from build123d import *

# Parameters (mm, degrees)
SZKIC1_W                    = 58
SZKIC1_H                    = 11
SZKIC1_R                    = 1.55
DODANIE_WYCI_GNI_CIE1_DEPTH = 6


with BuildPart() as part:
    # Szkic1 → Dodanie-wyciągnięcie1 (new body)
    with BuildSketch(Plane.ZY):
        with Locations((-846, 35.19227062)):
            Rectangle(SZKIC1_W, SZKIC1_H)
        with Locations((-869, 36.69227062)):
            Circle(SZKIC1_R, mode=Mode.SUBTRACT)
        with Locations((-821, 36.69227062)):
            Circle(SZKIC1_R, mode=Mode.SUBTRACT)
    extrude(amount=DODANIE_WYCI_GNI_CIE1_DEPTH)


solid = part.part
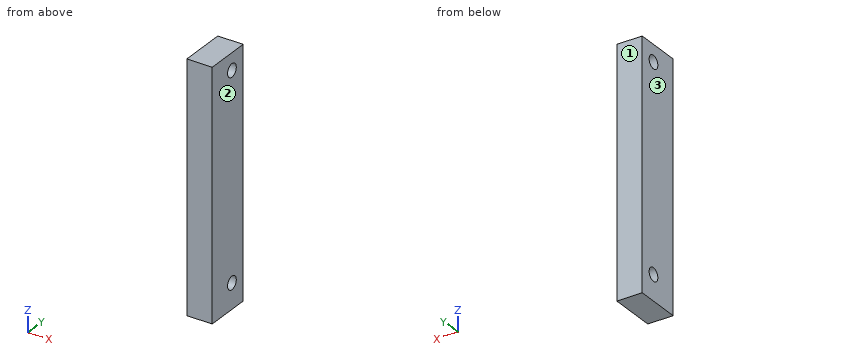
For this review, take the finished solid that the model builds, in its own axes (mm). Face numbers are marked on the shaded views. Round coordinates to 2 decimals unless told otherwise and drop trailing zeros. Order: outer loops, then holes, each group sorted by start corner. A loop starts at its lowest first (then second) coordinate and runs counter-clockwise, first axis right, second up. Notation, with made-up numbers: (63.25, -26) -> (84.25, -26) arc R21 cw to (84.25, -21) -> close; hole circle Ø6 at (36, 49.5). An arc over 180 degrees is marked (long way). Put each result on its own line as item: value.
Q1. Add section A-A on z = -869. Write out the cut boundary in (x, y), plus the area to 3 significant figures.
Check result:
outline: (-6, 29.69) -> (0, 29.69) -> (0, 35.14) -> (-6, 35.14) -> close; (-6, 38.24) -> (0, 38.24) -> (0, 40.69) -> (-6, 40.69) -> close
area: 47.4 mm2
Q2. Mouldability with a two-part tool opening along X and no side actions: class the marked faces 1, 2 and 3 as pulls with the +X half, pulls with the -X half, needs draft (parallel to the pull), parting line crosses it, or undercut.
Check result:
face 1: needs draft
face 2: pulls with the +X half
face 3: pulls with the -X half
Q3. For probe 1 along Y at (x, z) = (-1.9, -821); probe 2 along Z at (x, y) = (-2.95, 36.25); probe 3 along Y at (x, z) = (-1.75, -868), list the stretches that pass through material, from the lowest coordinate up. Write a range as [from, to].
Check result:
probe 1: [29.69, 35.14], [38.24, 40.69]
probe 2: [-875, -870.49], [-867.51, -822.49], [-819.51, -817]
probe 3: [29.69, 35.51], [37.88, 40.69]
Q4. Add section B-B on x = -2.15. Write out the cut boundary in (y, z), plus the area to 3 significant figures.
Check result:
outline: (29.69, -875) -> (40.69, -875) -> (40.69, -817) -> (29.69, -817) -> close; hole circle Ø3.1 at (36.69, -869); hole circle Ø3.1 at (36.69, -821)
area: 623 mm2
